Autodesk Inventor part; units mm, degrees
ref_plane "YZ Plane" through (0, 0, 0) normal (1, 0, 0) x (0, 1, 0)
ref_plane "XZ Plane" through (0, 0, 0) normal (0, 1, 0) x (-1, 0, 0)
ref_plane "XY Plane" through (0, 0, 0) normal (0, 0, 1) x (1, 0, 0)
sketch "Sketch1" plane through (0, 0, 0) normal (1, 0, 0) x (0, 1, 0)
  line L0 (0, 0) -> (40, 0)
  line L1 (40, 0) -> (40, -5)
  line L2 (40, -40) -> (5, -40) construction
  line L3 (0, -40) -> (0, 0)
  line L4 (40, 0) -> (40, -5)
  line L5 (40, -5) -> (5, -40)
  line L6 (0, -40) -> (5, -40)
  line L7 (40, -5) -> (5, -5)
  line L8 (5, -5) -> (5, -40)
  line L9 (40, -5) -> (40, -40) construction
  line L10 (5, -40) -> (0, -40)
  line L11 (37, 0) -> (35, 0)
  line L12 (35, 0) -> (35, 4.3)
  line L13 (35, 4.3) -> (37, 4.3)
  line L14 (37, 4.3) -> (37, 0)
  line L15 (6, 0) -> (4, 0)
  line L16 (4, 0) -> (4, 4.3)
  line L17 (4, 4.3) -> (6, 4.3)
  line L18 (6, 4.3) -> (6, 0)
  point P0 (5, 0)
  dimension "d0" = 40
  dimension "d1" = 5
  dimension "d2" = 2
  dimension "d3" = 4.3
  dimension "d4" = 4
  dimension "d5" = 3
extrude "Extrusion1" add sketch "Sketch1" along normal mid plane 40 contours L0 L1 L7 L8 L6 L3 | L8 L7 L5
extrude "Extrusion2" cut sketch "Sketch1" along normal mid plane 30 contours L8 L7 L5
extrude "Extrusion3" add sketch "Sketch1" along normal mid plane 8 contours L16 L17 L18 L0 | L12 L13 L14 L0
sketch "Sketch2" plane through (15, 5, -5) normal (0, 1, 0) x (-1, 0, 0)
  line L0 (15, -10) -> (15, -25) construction
  line L1 (10.5, -10) -> (10.5, -25)
  line L2 (19.5, -25) -> (19.5, -10)
  arc A0 (19.5, -10) -> (10.5, -10) centre (15, -10) ccw
  arc A1 (10.5, -25) -> (19.5, -25) centre (15, -25) ccw
  line L3 (30, 0) -> (0, 0)
  point P0 (15, 5)
  point P1 (15, -17.5)
  point P2 (15, 0)
  dimension "d12" = 15
  dimension "d13" = 9
  dimension "d14" = 10
extrude "Extrusion4" cut sketch "Sketch2" against normal through all
sketch "Sketch3" plane through (-15, 5, -5) normal (0, 0, -1) x (1, 0, 0)
  line L0 (-5, 5) -> (35, 5)
  circle A0 centre (15, -16) radius 4.5
  line L1 (0, -35) -> (30, -35)
  line L2 (15, -16) -> (15, -35) construction
  point P0 (15, 5)
  dimension "d18" = 9
  dimension "d21" = 19
extrude "Extrusion5" cut sketch "Sketch3" against normal through all
properties part number "Gusset_4040_8" material "Aluminum"
Design review of the part built by this model. Coordinates are the model's own, in mm. A direction names the side the tool comes from. Coordinates: 2 decimals unless noted, no trailing zeros. Write each loop counter-clockwise with the first axis right and the second up, starting at its lowest first coordinate (ties: lowest second). Pieces come first, ordered by that corner, then holes.
1) To check wall thickness, follow L1, parallel to Y at x = 0, z = -3.65; L2, parallel to X at y = 21, z = -3.5; L3, parallel to Y at x = 12, z = -28.5. State the ranges of each line that lie inside material, in increasing order.
2) Insertion check: pin 1 (1 mm diameter, centred on y = 5.5, z = 2.5, fed in from -X); pin 2 (6 mm diameter, centred on x = 10.5, y = 8.5, fed in from +Z); pin 3 (10 mm diameter, centred on x = 1, y = 16, fed in from -Z). Each pin has a flat end and moves straight along its axis. Give the tip position at first contact, or say it passes through.
3) Add section D-D (y = 14). Write out the cut boundary in (x, z).
4) Mouldability with a two-part tool opening along X and no side actions: class faces 4 (the flat face through (-4, 36, 2)), 5 (the flat face through (15, 18, -18)), 6 (the flat face through (-5, 20, 0)) as +X half, -X half, draft (parallel to the pull), parting line (faces both ways), or undercut.
5) Add section C-C (y = 21). Write out the cut boundary in (x, z).
6) Add section A-A (z = -21.5). Write out the cut boundary in (x, y), plus the area to 3 significant figures.
7) Add section B-B (x = 0). Write out the cut boundary in (y, z).
8) Machinability: for faces 1 (the flat face through (-4.5, 3, -23)), 2 (the flat face through (-4, 5, 2)), 3 (the flat face through (0, 27, -5)), which of the approach directions +Z, -Z, +X, -X, +Y, -Y give a long, thin tool a straight path to every point of the face, cutting with its end or side? Answer none if there is none.
Check result:
1. L1: y = 0 to 16.5, 25.5 to 40
1. L2: x = -20 to -4.5, 4.5 to 20
1. L3: y = 0 to 5
2. pin 1: stops at x = -4
2. pin 2: stops at z = 0
2. pin 3: stops at z = -5
3. outline: (-20, -31) - (-15, -31) - (-15, -5) - (15, -5) - (15, -31) - (20, -31) - (20, 0) - (-20, 0) - close
4. face 4: -X half
4. face 5: undercut
4. face 6: draft
5. outline: (-20, -24) - (-15, -24) - (-15, -5) - (-4.5, -5) - (-4.5, 0) - (-20, 0) - close; (4.5, -5) - (15, -5) - (15, -24) - (20, -24) - (20, 0) - (4.5, 0) - close
6. outline: (-20, 0) - (-4.5, 0) - (-4.5, 5) - (-15, 5) - (-15, 23.5) - (-20, 23.5) - close; (4.5, 0) - (20, 0) - (20, 23.5) - (15, 23.5) - (15, 5) - (4.5, 5) - close
6. area: 340 mm2
7. outline: (0, -40) - (5, -40) - (5, -34.5) - (0, -34.5) - close; (0, -10.5) - (5, -10.5) - (5, -5) - (16.5, -5) - (16.5, 0) - (6, 0) - (6, 4.3) - (4, 4.3) - (4, 0) - (0, 0) - close; (25.5, -5) - (40, -5) - (40, 0) - (37, 0) - (37, 4.3) - (35, 4.3) - (35, 0) - (25.5, 0) - close
8. face 1: +Y, -Y
8. face 2: +Z, -X, +Y, -Y
8. face 3: -Z, +Y
